For this review, take the finished solid that the model builds, in its own axes (mm). Round coordinates to 2 decimals unless told otherwise and drop trailing zeros. Write each loop counter-clockwise with the first axis right and the second up, starting at its lowest first coordinate (ties: lowest second). Pieces come first, ordered by that corner, then holes.
from build123d import *

# Parameters (mm, degrees)
SKETCH1_R           = 14.351
SKETCH1_R_2         = 2.54
SKETCH1_R_3         = 3.175
SKETCH1_R_4         = 1.27
BOSS_EXTRUDE1_DEPTH = 1.5875
SKETCH2_R           = 2.54
BOSS_EXTRUDE2_DEPTH = 1.5875
SKETCH3_R           = 2.54
CUT_EXTRUDE1_DEPTH  = 288.162032059


with BuildPart() as part:
    # Sketch1 → Boss-Extrude1 (new body)
    with BuildSketch(Plane.XY):
        with BuildLine():
            Line((88.9, 212.09), (88.9, 5.08))
            ThreePointArc((88.9, 5.08), (87.412102448, 1.487897552), (83.82, 0))
            Line((83.82, 0), (5.08, 0))
            ThreePointArc((5.08, 0), (1.487897552, 1.487897552), (0, 5.08))
            Line((0, 5.08), (0, 73.969993162))
            ThreePointArc((0, 73.969993162), (0.063384098, 74.769971217), (0.25195468, 75.549986324))
            Line((0.25195468, 75.549986324), (45.969223296, 215.249986324))
            ThreePointArc((45.969223296, 215.249986324), (49.662087504, 220.315906061), (55.625313935, 222.25))
            Line((55.625313935, 222.25), (78.74, 222.25))
            ThreePointArc((78.74, 222.25), (85.924204897, 219.274204897), (88.9, 212.09))
        make_face()
        with Locations((68.199, 201.93)):
            Circle(SKETCH1_R, mode=Mode.SUBTRACT)
        with Locations((68.199, 100.838)):
            Circle(SKETCH1_R, mode=Mode.SUBTRACT)
        with Locations((68.199, 144.78)):
            Circle(SKETCH1_R_2, mode=Mode.SUBTRACT)
        with Locations((68.199, 46.99)):
            Circle(SKETCH1_R_2, mode=Mode.SUBTRACT)
        with Locations((27.94, 46.99)):
            Circle(SKETCH1_R, mode=Mode.SUBTRACT)
        with Locations((6.35, 9.652)):
            Circle(SKETCH1_R_3, mode=Mode.SUBTRACT)
        with Locations((31.75, 9.652)):
            Circle(SKETCH1_R_3, mode=Mode.SUBTRACT)
        with Locations((57.15, 9.652)):
            Circle(SKETCH1_R_3, mode=Mode.SUBTRACT)
        with Locations((82.55, 9.652)):
            Circle(SKETCH1_R_3, mode=Mode.SUBTRACT)
        with Locations(Location((69.85, 22.352, 0), (0, 0, 180))):
            Circle(SKETCH1_R_3, mode=Mode.SUBTRACT)
        with Locations(Location((44.45, 21.844, 0), (0, 0, 180))):
            Circle(SKETCH1_R_3, mode=Mode.SUBTRACT)
        with Locations(Location((19.05, 21.844, 0), (0, 0, 180))):
            Circle(SKETCH1_R_3, mode=Mode.SUBTRACT)
        with Locations((46.228, 46.99)):
            Circle(SKETCH1_R_4, mode=Mode.SUBTRACT)
        with Locations((37.084, 31.152127416)):
            Circle(SKETCH1_R_4, mode=Mode.SUBTRACT)
        with Locations((18.796, 31.152127416)):
            Circle(SKETCH1_R_4, mode=Mode.SUBTRACT)
        with Locations((9.652, 46.99)):
            Circle(SKETCH1_R_4, mode=Mode.SUBTRACT)
        with Locations((18.796, 62.827872584)):
            Circle(SKETCH1_R_4, mode=Mode.SUBTRACT)
        with Locations((37.084, 62.827872584)):
            Circle(SKETCH1_R_4, mode=Mode.SUBTRACT)
    extrude(amount=BOSS_EXTRUDE1_DEPTH)

    # Sketch2 → Boss-Extrude2 (add)
    with BuildSketch(Plane.XY.offset(1.5875)):
        with BuildLine():
            Line((45.969223296, 215.249986324), (62.593684611, 266.049986324))
            ThreePointArc((62.593684611, 266.049986324), (66.286548819, 271.115906061), (72.24977525, 273.05))
            Line((72.24977525, 273.05), (78.74, 273.05))
            ThreePointArc((78.74, 273.05), (85.924204897, 270.074204897), (88.9, 262.89))
            Line((88.9, 262.89), (88.9, 212.09))
            Line((88.9, 212.09), (78.74, 222.25))
            Line((78.74, 222.25), (55.625313935, 222.25))
            Line((55.625313935, 222.25), (45.969223296, 215.249986324))
        make_face()
        with Locations((76.2, 260.35)):
            Circle(SKETCH2_R, mode=Mode.SUBTRACT)
    extrude(amount=-BOSS_EXTRUDE2_DEPTH)

    # Sketch3 → Cut-Extrude1 (cut, through all)
    with BuildSketch(Plane.XY.offset(1.5875)):
        with Locations((17.78, 83.058)):
            Circle(SKETCH3_R)
    extrude(amount=-CUT_EXTRUDE1_DEPTH, mode=Mode.SUBTRACT)


solid = part.part
(1) We need section C-C, the plane y = 260.35. Give the boundary of the cut face in (x, z), and give its area (3 significant figures).
Geometry check:
outline: (60.73, 0) - (73.66, 0) - (73.66, 1.59) - (60.73, 1.59) - close; (78.74, 0) - (88.9, 0) - (88.9, 1.59) - (78.74, 1.59) - close
area: 36.7 mm2
(2) We need section A-A, the plane y = 199. Give the boundary of the cut face in (x, z), and give its area (3 significant figures).
Geometry check:
outline: (40.65, 0) - (54.15, 0) - (54.15, 1.59) - (40.65, 1.59) - close; (82.25, 0) - (88.9, 0) - (88.9, 1.59) - (82.25, 1.59) - close
area: 32.0 mm2
(3) For line 1 along Y through (x, z) = (69.85, 0.8); line 2 along X through (y, z) = (105, 0.35); line 3 along X through (y, z) = (84.5, 0.1), list the stretches that pass through material, from the lowest coordinate up.
Geometry check:
line 1: y = 0 to 19.18, 25.53 to 45.06, 48.92 to 86.58, 115.09 to 142.85, 146.71 to 187.67, 216.19 to 272.76
line 2: x = 9.89 to 54.46, 81.93 to 88.9
line 3: x = 3.18 to 15.69, 19.87 to 88.9
(4) We need section D-D, the plane y = 160. Give the boundary of the cut face in (x, z).
Geometry check:
outline: (27.89, 0) - (88.9, 0) - (88.9, 1.59) - (27.89, 1.59) - close
(5) Mouldability with a two-part tool opening along Y and no side actions: class faces 1 (the face through (1.528, 1.449, 0.783)), 2 (the face through (85.578, 10.606, 0.783)), 3 (the face through (66.21, 271.06, 0.8)) as pulls with the +Y half, pulls with the -Y half, needs draft (parallel to the pull), parting line crosses it, or undercut.
Geometry check:
face 1: pulls with the -Y half
face 2: undercut
face 3: pulls with the +Y half
(6) We need section B-B, the plane z = 1.15. State how many separate pieces and enclosed holes the cut face has, and give its area (3 significant figures).
Geometry check:
separate pieces: 1
enclosed holes: 20
area: 15,500 mm2
